```python
from build123d import *

# Parameters (mm, degrees)
SKETCH1_W           = 12.1
SKETCH1_H           = 6
BOSS_EXTRUDE1_DEPTH = 2.5
SKETCH2_R           = 2.75
SKETCH2_R_2         = 1.8
BOSS_EXTRUDE2_DEPTH = 2
SKETCH3_R           = 0.6
BOSS_EXTRUDE3_DEPTH = 0.8
FILLET1_R           = 0.2
SKETCH4_W           = 1
SKETCH4_H           = 2.460309858
SKETCH4_H_2         = 2.047502849
BOSS_EXTRUDE4_DEPTH = 0.2


with BuildPart() as part:
    # Sketch1 → Boss-Extrude1 (new body, symmetric)
    with BuildSketch(Plane(origin=(0, 0, 0), x_dir=(1, 0, 0), z_dir=(0, 1, 0))):
        Rectangle(SKETCH1_W, SKETCH1_H)
    extrude(amount=BOSS_EXTRUDE1_DEPTH, both=True)

    # Sketch2 → Boss-Extrude2 (add)
    with BuildSketch(Plane.ZY.offset(6.05)):
        Circle(SKETCH2_R)
        Circle(SKETCH2_R_2, mode=Mode.SUBTRACT)
    extrude(amount=BOSS_EXTRUDE2_DEPTH)

    # Sketch3 → Boss-Extrude3 (add)
    with BuildSketch(Plane.XZ.offset(2.5)):
        with Locations((-4.25, 0)):
            Circle(SKETCH3_R)
        with Locations((2.75, 0)):
            Circle(SKETCH3_R)
    extrude(amount=BOSS_EXTRUDE3_DEPTH)

    # Fillet1
    fillet1_edges = [part.edges().sort_by_distance(p)[0] for p in [
        (-4.85, -3.3, 0),
        (2.15, -3.3, 0),
    ]]
    fillet(fillet1_edges, radius=FILLET1_R)

    # Sketch4 → Boss-Extrude4 (add)
    with BuildSketch(Plane.XZ.offset(2.5)):
        with Locations((-2.95, -2.769845071)):
            Rectangle(SKETCH4_W, SKETCH4_H)
        with Locations((0.05, -2.769845071)):
            Rectangle(SKETCH4_W, SKETCH4_H)
        with Locations((4.05, -2.769845071)):
            Rectangle(SKETCH4_W, SKETCH4_H)
        with Locations((5.55, 2.976248576)):
            Rectangle(SKETCH4_W, SKETCH4_H_2)
    extrude(amount=BOSS_EXTRUDE4_DEPTH)


solid = part.part
```
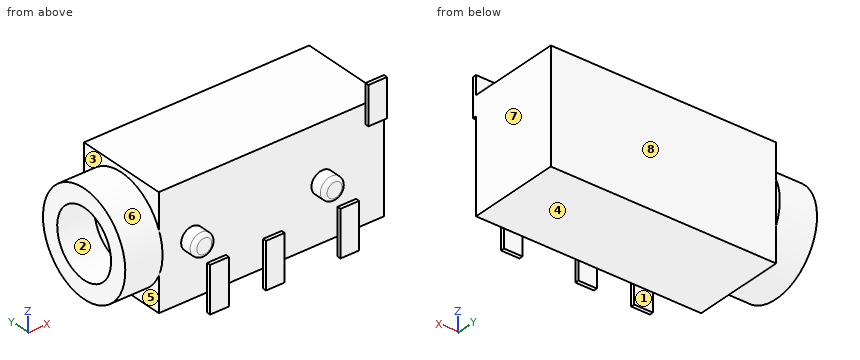
Here's how the part is built. I have some questions about the finished solid (model axes, mm). Face numbers are marked on the shaded views. A direction names the side the tool comes from. Round coordinates to 2 decimals unless told otherwise and drop trailing zeros. Write each loop counter-clockwise with the first axis right and the second up, starting at its lowest first coordinate (ties: lowest second). Pieces come first, ordered by that corner, then holes.
Q1. If we mould it in two halves opening along Y, with no side actions, what happens to the marked faces 1, 2 and 3? For each: +Y half, -Y half, draft (parallel to the pull), parting line (faces both ways), or undercut.
Q2. If we section it at A-A on z = -3.5: Write out the boundary of the cut face in (x, y).
Q3. If we section it at D-D on y = 0: Write out the boundary of the cut face in (x, z).
Q4. If we section it at C-C on z = 2.5: Write out the boundary of the cut face in (x, y), plus the area to 3 significant figures.
Q5. Will these pins go through, and if not, where does the flat tip stop? P1, Ø1.1, axis at x = 0, z = -2.5, coming from the -Y side; P2, Ø3, axis at x = 2, z = -0.5, coming from the -Y side; P3, Ø1.5, axis at x = -2.5, y = 1, coming from the -Z side; P4, Ø1.1, axis at x = 0, z = -3.5, coming from the +Y side.
Q6. Which directions (+Z, -Z, +X, -X, +Y, -Y) give clear straight access to the entire face, cutting with the end or side of a thin tool? Please do the marked faces 4, 5, 6, 7 and 8.
Q7. Please list where these lines run through material, in increasing order: probe 1 along Y at (x, z) = (-6.7, 0); probe 2 along X at (y, z) = (-1.75, 2.25); probe 3 along Y at (x, z) = (-4.25, -1.25).
Q8. If we section it at B-B on x = -0.25: Write out the boundary of the cut face in (y, z).
Answer below:
1. face 1: +Y half
1. face 2: undercut
1. face 3: draft
2. outline: (-3.45, -2.7) - (-2.45, -2.7) - (-2.45, -2.5) - (-3.45, -2.5) - close; (-0.45, -2.7) - (0.55, -2.7) - (0.55, -2.5) - (-0.45, -2.5) - close; (3.55, -2.7) - (4.55, -2.7) - (4.55, -2.5) - (3.55, -2.5) - close
3. outline: (-8.05, -2.75) - (-6.05, -2.75) - (-6.05, -3) - (6.05, -3) - (6.05, 3) - (-6.05, 3) - (-6.05, 2.75) - (-8.05, 2.75) - (-8.05, 1.8) - (-6.05, 1.8) - (-6.05, -1.8) - (-8.05, -1.8) - close
4. outline: (-8.05, -1.15) - (-6.05, -1.15) - (-6.05, -2.5) - (5.05, -2.5) - (5.05, -2.7) - (6.05, -2.7) - (6.05, 2.5) - (-6.05, 2.5) - (-6.05, 1.15) - (-8.05, 1.15) - close
4. area: 65.3 mm2
5. P1: stops at y = -2.7
5. P2: stops at y = -3.3
5. P3: stops at z = -3
5. P4: stops at y = 2.5
6. face 4: -Z, +X, -X, +Y
6. face 5: -Z, -X
6. face 6: -X
6. face 7: +Z, -Z, +X, +Y, -Y
6. face 8: +Z, -Z, +X, +Y
7. probe 1: y = -2.75 to -1.8, 1.8 to 2.75
7. probe 2: x = -6.05 to 6.05
7. probe 3: y = -2.5 to 2.5
8. outline: (-2.7, -4) - (-2.5, -4) - (-2.5, -3) - (2.5, -3) - (2.5, 3) - (-2.5, 3) - (-2.5, -1.54) - (-2.7, -1.54) - close
